Autodesk Inventor part; units mm, degrees
ref_plane "YZ Plane" through (0, 0, 0) normal (1, 0, 0) x (0, 1, 0)
ref_plane "XZ Plane" through (0, 0, 0) normal (0, 1, 0) x (-1, 0, 0)
ref_plane "XY Plane" through (0, 0, 0) normal (0, 0, 1) x (1, 0, 0)
sketch "Sketch1" plane through (0, 0, 0) normal (0, 1, 0) x (-1, 0, 0)
  line L0 (0, 0) -> (0, 12.8)
  line L1 (0, 12.8) -> (-2, 12.8)
  line L2 (-2, 12.8) -> (-2, 9.4)
  line L3 (-3, 7.8) -> (-3, 2.8)
  line L4 (-3, 2.8) -> (-5, 2.8)
  line L5 (-5, 2.8) -> (-5, 0)
  line L6 (-5, 0) -> (0, 0)
  line L7 (-1.6, 9) -> (-1.6, 7.8)
  line L8 (-3, 7.8) -> (-1.6, 7.8)
  line L9 (-1.6, 9) -> (-2, 9.4)
  dimension "d0" = 10
  dimension "d1" = 6
  dimension "d2" = 4
  dimension "d4" = 5
  dimension "d5" = 2.8
  dimension "d15" = 5
  dimension "d16" = 3.2
  dimension "d17" = 1.2
  dimension "d18" = 45
revolve "Revolution1" add sketch "Sketch1" angle 360 about axis through (0, 0, 0) along (0, 0, 1)
thread "Thread1"
sketch "Sketch2" plane through (0, 0, 0) normal (0, 0, -1) x (-1, 0, 0)
  line L0 (0, 1.4434) -> (1.25, 0.7217)
  line L1 (1.25, 0.7217) -> (1.25, -0.7217)
  line L2 (1.25, -0.7217) -> (0, -1.4434)
  line L3 (0, -1.4434) -> (-1.25, -0.7217)
  line L4 (-1.25, -0.7217) -> (-1.25, 0.7217)
  line L5 (-1.25, 0.7217) -> (0, 1.4434)
  point P0 (0, 0)
  point P1 (0, 0)
  dimension "d9" = 2.5
extrude "Extrusion1" cut sketch "Sketch2" against normal blind 2
chamfer "Chamfer1" distance 0.43 angle 45 1 edges at (-2, 0, 12.8)
properties part number "DBTSY4-5-5-DHC-PC" material "Stainless Steel AISI 304"
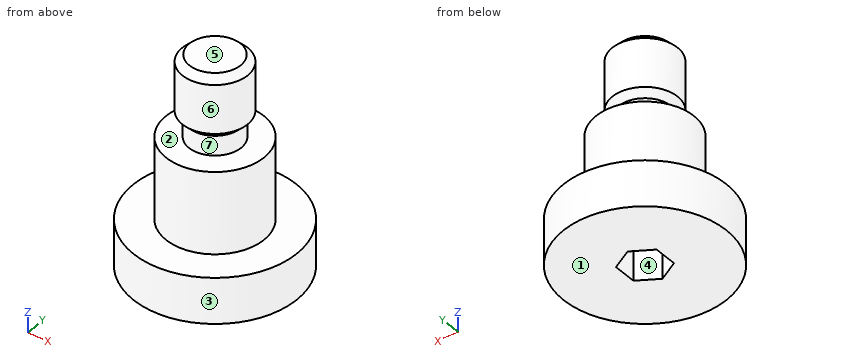
Read the model definition and answer for the solid it produces. Units are mm, in the model's axes. Face numbers are marked on the shaded views. A direction names the side the tool comes from. Coordinates: 2 decimals unless noted, no trailing zeros. Write each loop counter-clockwise with the first axis right and the second up, starting at its lowest first coordinate (ties: lowest second). Pieces come first, ordered by that corner, then holes. Notation, with made-up numbers: (-15.5, 87.5) -> (38.5, 87.5) arc R15 cw to (38.5, 93.5) -> close; hole circle Ø2 at (50, 13.5). An arc over 180 degrees is marked (long way). Answer as a JSON object with one key per item and string values.
Q1. Determine the mould class of the marked faces 1, 2 and 3 for opening direction Z: pulls with the +Z half, pulls with the -Z half, needs draft (parallel to the pull), parting line crosses it, or undercut.
The answers:
{"face 1": "pulls with the -Z half", "face 2": "undercut", "face 3": "needs draft"}
Q2. Consider line 1 (Z direction, x = -2.25, y = -1.5); line 2 (Z direction, x = 4, y = -2.75); line 3 (X direction, y = 1, z = 1.5). Determine where each line is inside the solid, lowest interval first. Write a range as [from, to].
The answers:
{"line 1": "z = [0, 7.8]", "line 2": "z = [0, 2.8]", "line 3": "x = [-4.9, -0.77], [0.77, 4.9]"}
Q3. A tool of negligible diameter and unlimited length cuts with its end or side. For the marked faces 4, 5, 6 and 7, from which of +Z, -Z, +X, -X, +Y, -Y can it reach the whole face along a straight path? Write none if from no direction.
The answers:
{"face 4": "-Z", "face 5": "+Z, +X, -X, +Y, -Y", "face 6": "+Z", "face 7": "none"}
Q4. The part is cut by section B-B on y = 2.75. Give the vertices of the cut face in (x, z).
The answers:
{"outline": "(-4.18, 0) -> (4.18, 0) -> (4.18, 2.8) -> (1.2, 2.8) -> (1.2, 7.8) -> (-1.2, 7.8) -> (-1.2, 2.8) -> (-4.18, 2.8) -> close"}
Q5. The part is cut by section C-C on z = 8.75. Give the vertices of the cut face in (x, y), then the cut area to 3 significant figures.
The answers:
{"outline": "circle Ø3.2 at (0, 0)", "area": "8.04 mm2"}
Q6. The part is cut by section A-A on z = 1.25. Give the vertices of the cut face in (x, y).
The answers:
{"outline": "circle Ø10 at (0, 0); hole (-1.25, -0.72) -> (0, -1.44) -> (1.25, -0.72) -> (1.25, 0.72) -> (0, 1.44) -> (-1.25, 0.72) -> close"}
Q7. Flat-ended cylindrical pins translate along their axes: pin 1 Ø1.3 at (x, y) = (-0.5, 0.5) entering from -Z; pin 2 Ø1.5 at (y, z) = (-2.5, 9.5) entering from +X; pin 3 Ø4 at (x, z) = (1, 6.5) entering from -Y; pin 4 Ø1 at (y, z) = (1, 1.5) entering from +X. Find the tip coordinate at first contact, or state that the pin passes through.
The answers:
{"pin 1": "stops at z = 0", "pin 2": "stops at x = 0.97", "pin 3": "stops at y = -3", "pin 4": "stops at x = 4.97"}
